CAD build for the part. Positions are in the model's coordinates, mm. Give positions to 0.01 mm unless a question says otherwise; leave off trailing zeros. Write each loop counter-clockwise with the first axis right and the second up, starting at its lowest first coordinate (ties: lowest second). Pieces come first, ordered by that corner, then holes. Notation, with made-up numbers: (15.25, 71.5) - (23.25, 71.5) arc R29 cw to (23.25, 104.5) - close; hole circle Ø8 at (9, 89.5). An arc over 180 degrees is marked (long way). Put each result on its own line as item: value. Start each with the question number.
1. Drop a flat-ended pin along its axis: pin 1 (6.5 mm diameter, centred on x = -157.5, z = 0, fed in from +Y). Give the stop position or say it passes through.
2. Cut at A-A on y = 1.5. List the corners of the cut face in (x, z).
3. Wall check: line 1 (Z direction, x = -157.5, y = 1); line 2 (X direction, y = 0.9, z = 3.5); line 3 (X direction, y = 0.7, z = -5.25). Give the ranges that are in metal, low to high.
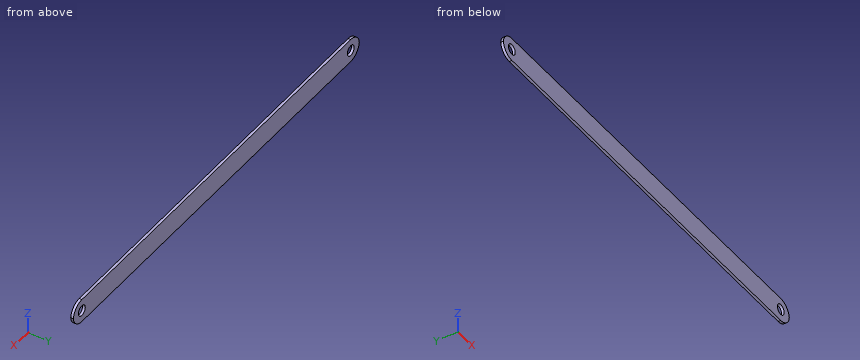
Autodesk Inventor part; units mm, degrees
ref_plane "YZ Plane" through (0, 0, 0) normal (1, 0, 0) x (0, 1, 0)
ref_plane "XZ Plane" through (0, 0, 0) normal (0, 1, 0) x (-1, 0, 0)
ref_plane "XY Plane" through (0, 0, 0) normal (0, 0, 1) x (1, 0, 0)
sketch "Boceto1" plane through (0, 0, 0) normal (0, 1, 0) x (-1, 0, 0)
  line L0 (385.7227, 0) -> (-335.8409, 0) construction
  line L1 (0, 516.0097) -> (0, -537.3218) construction
  line L2 (-157.5, -9) -> (157.5, -9)
  line L3 (167.5, 1) -> (167.5, -1)
  line L4 (157.5, 9) -> (-157.5, 9)
  line L5 (-167.5, -1) -> (-167.5, 1)
  line L6 (-167.5, -9) -> (167.5, 9) construction
  line L7 (167.5, -9) -> (-167.5, 9) construction
  arc A0 (167.5, -1) -> (157.5, 9) centre (157.5, -1) ccw
  arc A1 (157.5, -9) -> (167.5, 1) centre (157.5, 1) ccw
  arc A2 (-167.5, 1) -> (-157.5, -9) centre (-157.5, 1) ccw
  arc A3 (-157.5, 9) -> (-167.5, -1) centre (-157.5, -1) ccw
  line L8 (157.5, 9) -> (157.5, -15.4925) construction
  circle A4 centre (157.5, 0) radius 4
  line L9 (-157.5, -9) -> (-157.5, 29.1929) construction
  circle A5 centre (-157.5, 0) radius 4
  point P0 (0, 0)
  point P1 (167.4499, 0)
  point P2 (-167.4499, 0)
  dimension "d0" = 18
  dimension "d1" = 335
  dimension "d2" = 10
  dimension "d3" = 8
  dimension "d4" = 8
extrude "Extrusión1" add sketch "Boceto1" along normal blind 2 contours A2 A3 L4 A0 A1 L2
Report:
1. pin 1: passes through
2. outline: (-167.45, 0) arc R10 ccw to (-157.5, -9) - (157.5, -9) arc R10 ccw to (167.45, 0) arc R10 ccw to (157.5, 9) - (-157.5, 9) arc R10 ccw to start; hole circle Ø8 at (-157.5, 0); hole circle Ø8 at (157.5, 0)
3. line 1: z = -9 to -4, 4 to 9
3. line 2: x = -166.43 to -159.44, -155.56 to 155.56, 159.44 to 166.43
3. line 3: x = -165.31 to 165.31
